```python
from build123d import *

# Parameters (mm, degrees)
F1_DEPTH = 21
F2_R     = 1.482571
F3_DEPTH = 6.001


with BuildPart() as f1:
    # F0 (on Top) → F1 (new body)
    with BuildSketch(Plane.XY):
        with BuildLine():
            ThreePointArc((25, 22.307473), (24.982152, 21.362986), (24.928635, 20.419847))
            Line((24.928635, 20.419847), (24.928635, 0))
            Line((24.928635, 0), (28, 0))
            Line((28, 0), (44, 0))
            Line((44, 0), (44, 6))
            Line((44, 6), (30.651433, 6))
            Line((30.651433, 6), (29.325717, 8.401437))
            Line((29.325717, 8.401437), (29.325717, 27.943285))
            Line((29.325717, 27.943285), (23.699379, 41.248079))
            Line((23.699379, 41.248079), (10.514447, 50.237805))
            Line((10.514447, 50.237805), (0, 52.635066))
            Line((0, 52.635066), (-10.514447, 50.237805))
            Line((-10.514447, 50.237805), (-23.699379, 41.248079))
            Line((-23.699379, 41.248079), (-29.325717, 27.943285))
            Line((-29.325717, 27.943285), (-29.325717, 8.401437))
            Line((-29.325717, 8.401437), (-30.651433, 6))
            Line((-30.651433, 6), (-44, 6))
            Line((-44, 6), (-44, 0))
            Line((-44, 0), (-28, 0))
            Line((-28, 0), (-24.928635, 0))
            Line((-24.928635, 0), (-24.928635, 20.419847))
            ThreePointArc((-24.928635, 20.419847), (-24.982152, 21.362986), (-25, 22.307473))
            ThreePointArc((-25, 22.307473), (0, 47.307473), (25, 22.307473))
        make_face()
    extrude(amount=F1_DEPTH)

    # F2 (on face) → F3 (cut, through all)
    with BuildSketch(Plane(origin=(0, 6, 0), x_dir=(-1, 0, 0), z_dir=(0, 1, 0))):
        with Locations((-37.325717, 10.5)):
            Circle(F2_R)
        with Locations((37.325717, 10.5)):
            Circle(F2_R)
    extrude(amount=-F3_DEPTH, mode=Mode.SUBTRACT)


solid = f1.part
```
Can you work these out from the model? Positions are in its coordinate system, mm. A direction names the side the tool comes from. Round coordinates to 2 decimals unless told otherwise and drop trailing zeros. Order: outer loops, then holes, each group sorted by start corner. A loop starts at its lowest first (then second) coordinate and runs counter-clockwise, first axis right, second up. Notation, with made-up numbers: (78, 5.5) -> (131, 5.5) arc R4 ccw to (131, 12.5) -> close; hole circle Ø9 at (14.25, 51). An arc over 180 degrees is marked (long way). Return JSON: item names as keys, results as strings. Group by question number.
1. If we section it at B-B, the plane y = 39: Write out the boundary of the cut face in (x, z).
2. We'd pull the mould along X, two halves only. Please class faces 1 (the face through (30, 7.18, 10.35)), 2 (the face through (24.929, 10, 10)), 3 (the face through (-5.184, 51.453, 10.353)): released by +X, released by -X, zero draft, split by the parting line, or undercut.
3. If we section it at C-C, the plane z = 14.75: Write out the boundary of the cut face in (x, y).
4. If we section it at A-A, the plane z = 10.5: Count the separate pieces of the cut face and the enclosed holes in it, then the cut area to 3 significant figures.
5. I need wall thicknesses on line 1 (X direction, y = 12.5, z = 3.5); line 2 (Y direction, x = -39, z = 6.75); line 3 (X direction, y = 3.5, z = 15). Which ranges of each line are inside material? Lowest first, please. Write a range as [from, to].
6. Which directions (+Z, -Z, +X, -X, +Y, -Y) give clear straight access to the entire face, cutting with the end or side of a thin tool? Please do faces 4 (the face through (-29.326, 18, 10)), 5 (the face through (39, 6, 10)), 6 (the face through (-35, 0, 10)).
7. If we section it at D-D, the plane x = 21: Write out the boundary of the cut face in (y, z), then the cut area to 3 significant figures.
8. Will these pins go through, and if not, where does the flat tip stop? pin 1 (8 mm diameter, centred on y = 18.5, z = 12.5, fed in from -X); pin 2 (10 mm diameter, centred on x = 34.5, z = 11, fed in from +Y); pin 3 (4 mm diameter, centred on y = 8.5, z = 2.5, fed in from +X).
Output values:
{
 "1": {"outline": "(-24.65, 0) -> (-18.61, 0) -> (-18.61, 21) -> (-24.65, 21) -> close; (18.61, 0) -> (24.65, 0) -> (24.65, 21) -> (18.61, 21) -> close"},
 "2": {"face 1": "released by +X", "face 2": "undercut", "face 3": "released by -X"},
 "3": {"outline": "(-44, 0) -> (-24.93, 0) -> (-24.93, 20.42) arc R25 cw to (-25, 22.31) arc R25 cw to (25, 22.31) arc R25 cw to (24.93, 20.42) -> (24.93, 0) -> (44, 0) -> (44, 6) -> (30.65, 6) -> (29.33, 8.4) -> (29.33, 27.94) -> (23.7, 41.25) -> (10.51, 50.24) -> (0, 52.64) -> (-10.51, 50.24) -> (-23.7, 41.25) -> (-29.33, 27.94) -> (-29.33, 8.4) -> (-30.65, 6) -> (-44, 6) -> close"},
 "4": {"separate pieces": "3", "enclosed holes": "0", "area": "727 mm²"},
 "5": {"line 1": "[-29.33, -24.93], [24.93, 29.33]", "line 2": "[0, 6]", "line 3": "[-44, -24.93], [24.93, 44]"},
 "6": {"face 4": "+Z, -Z, -X, +Y", "face 5": "+Z, -Z, +X, +Y", "face 6": "+Z, -Z, +X, -X, -Y"},
 "7": {"outline": "(35.87, 0) -> (43.09, 0) -> (43.09, 21) -> (35.87, 21) -> close", "area": "152 mm²"},
 "8": {"pin 1": "x = -29.33", "pin 2": "y = 8.09", "pin 3": "x = 30.38"}
}
